Can you work these out from the model? Positions are in its coordinate system, mm. A direction names the side the tool comes from. Give positions to 0.01 mm unless a question says otherwise; leave off trailing zeros. Order: outer loops, then holes, each group sorted by start corner. A loop starts at its lowest first (then second) coordinate and runs counter-clockwise, first axis right, second up. Notation, with made-up numbers: (24, 63.25) - (28, 63.25) arc R28 ccw to (28, 88.25) - close; hole circle Ø7 at (86, 62.5). An arc over 180 degrees is marked (long way). Answer as a JSON object with one key per item and string values.
```python
from build123d import *

# Parameters (mm, degrees)
F0_R     = 22
F1_DEPTH = 32.5
F2_R     = 3
F3_DEPTH = 18
F4_R     = 1
F5_DEPTH = 4
F9_DEPTH = 20
F10_SIZE = 0.5


with BuildPart() as f1:
    # F0 (on Right) → F1 (new body, symmetric)
    with BuildSketch(Plane.YZ):
        Circle(F0_R)
    extrude(amount=F1_DEPTH, both=True)

    # F2 (on face) → F3 (join)
    with BuildSketch(Plane.YZ.offset(32.5)):
        Circle(F2_R)
    extrude(amount=F3_DEPTH)

    # F4 (on face) → F5 (cut)
    with BuildSketch(Plane.YZ.offset(32.5)):
        with Locations((0, 15)):
            Circle(F4_R)
        with Locations((-15, 0)):
            Circle(F4_R)
        with Locations((0, -15)):
            Circle(F4_R)
        with Locations((15, 0)):
            Circle(F4_R)
        with Locations((-8.838835, 8.838835)):
            Circle(F4_R)
        with Locations((-8.838835, -8.838835)):
            Circle(F4_R)
        with Locations((8.838835, -8.838835)):
            Circle(F4_R)
        with Locations((8.838835, 8.838835)):
            Circle(F4_R)
    extrude(amount=-F5_DEPTH, mode=Mode.SUBTRACT)

    # F6 (on Front) → F7 (revolve, cut)
    with BuildSketch(Plane.XZ):
        Polygon((-32.5, 6), (-32.5, 3), (-31, 3), (-31, 3.5), (-30.5, 3.5), (-30.5, 6), align=None)
    revolve(axis=Axis((7.880477, 0, 0), (1, 0, 0)), mode=Mode.SUBTRACT)

    # F8 (on face) → F9 (join)
    with BuildSketch(Plane(origin=(-32.5, 0, 0), x_dir=(0, -1, 0), z_dir=(-1, 0, 0))):
        with BuildLine():
            ThreePointArc((-3.473684, -21.724031), (0, -22), (3.473684, -21.724031))
            ThreePointArc((3.473684, -21.724031), (5.962368, -18.287979), (2.526316, -15.799295))
            ThreePointArc((2.526316, -15.799295), (0, -16), (-2.526316, -15.799295))
            ThreePointArc((-2.526316, -15.799295), (-5.962368, -18.287979), (-3.473684, -21.724031))
        make_face()
    extrude(amount=F9_DEPTH)

    # F10
    f10_edges = [f1.edges().sort_by_distance(p)[0] for p in [
        (50.5, -3, 0),
    ]]
    chamfer(f10_edges, length=F10_SIZE)


solid = f1.part
```
Q1. If we section it at C-C, the plane x = 25: Please give me the cut outline in (y, z), then the cut area to 3 significant figures.
Recorded:
{"outline": "circle Ø44 at (0, 0)", "area": "1,520 mm^2"}
Q2. I need wall thicknesses on L1, parallel to X at y = 19, z = 4; L2, parallel to X at y = -9, z = -8.5; L3, parallel to Z at x = 29, y = 15. Which ranges of each line are inside material? Lowest first, please.
Recorded:
{"L1": "x = -32.5 to 32.5", "L2": "x = -32.5 to 28.5", "L3": "z = -16.09 to -1, 1 to 16.09"}
Q3. We'd pull the mould along Z, two halves only. Please class faces 4 (the face through (-42.36, 5.95, -18.22)), 5 (the face through (28.5, -9, 9)), 6 (the face through (-32.5, 5, 5)): released by +Z, released by -Z, zero draft, split by the parting line, or undercut.
Recorded:
{"face 4": "split by the parting line", "face 5": "undercut", "face 6": "zero draft"}
Q4. If we section it at D-D, the plane y = -15: Please give me the cut outline in (x, z).
Recorded:
{"outline": "(-32.5, -16.09) - (32.5, -16.09) - (32.5, -1) - (28.5, -1) - (28.5, 1) - (32.5, 1) - (32.5, 16.09) - (-32.5, 16.09) - close"}
Q5. I'm going to push flat-ended pins straight in: pin 1 Ø2.5 at (y, z) = (15, 0) entering from -X; pin 2 Ø1 at (y, z) = (-6, 5.5) entering from +X; pin 3 Ø0.6 at (y, z) = (9, 9) entering from +X. Where does each tip first touch, or does it pass through?
Recorded:
{"pin 1": "stops at x = -32.5", "pin 2": "stops at x = 32.5", "pin 3": "stops at x = 28.5"}
Q6. Which directions (+Z, -Z, +X, -X, +Y, -Y) give clear straight access to the entire face, cutting with the end or side of a thin tool? Please do faces 1 (the face through (50.5, 0, 0)), 2 (the face through (-30.746, 1.341, 3.233)), 3 (the face through (30.53, 9.3, 7.95)).
Recorded:
{"face 1": "+Z, -Z, +X, +Y, -Y", "face 2": "-X", "face 3": "+X"}
